```python
from build123d import *

# Parameters (mm, degrees)
CUT_EXTRUDE1_DEPTH       = 13.7
FILLET1_R                = 4
CIRPATTERN4_COUNT        = 6
FILLET1_OF_CIRPATTERN4_R = 4
CHAMFER1_SIZE            = 1
SKETCH9_R                = 83.55
SKETCH9_R_2              = 82.55
BOSS_EXTRUDE1_DEPTH      = 12.7


with BuildPart() as part:
    # Sketch2 → Revolve1 (revolve)
    with BuildSketch(Plane(origin=(0, 0, 0), x_dir=(0, 0, -1), z_dir=(1, 0, 0))):
        Polygon((-39.2125, 0), (-82.55, 0), (-82.55, 12.7), (-49.2125, 12.7), (-49.2125, 10), (-39.2125, 10), align=None)
    revolve(axis=Axis((0, -0.9525, 0), (0, 1, 0)))

    # Sketch8 → Cut-Extrude1 (cut, through all)
    with BuildSketch(Plane(origin=(0, 12.7, 0), x_dir=(1, 0, 0), z_dir=(0, 1, 0))):
        with BuildLine():
            Line((-34.364196, 69.520533), (-22.66059, 49.249293))
            ThreePointArc((-22.66059, 49.249293), (0, 54.2125), (22.66059, 49.249293))
            Line((22.66059, 49.249293), (34.364196, 69.520533))
            ThreePointArc((34.364196, 69.520533), (0, 77.55), (-34.364196, 69.520533))
        make_face()
    cut_extrude1 = extrude(amount=-CUT_EXTRUDE1_DEPTH, mode=Mode.SUBTRACT)

    # Fillet1
    fillet1_edges = [part.edges().sort_by_distance(p)[0] for p in [
        (22.66059, 6.35, -49.249293),
        (-22.66059, 6.35, -49.249293),
        (-34.364196, 6.35, -69.520533),
        (34.364196, 6.35, -69.520533),
    ]]
    fillet(fillet1_edges, radius=FILLET1_R)

    # CirPattern4: Cut-Extrude1 ×6 about axis
    cirpattern4_axis = Axis((0, 0, 0), (0, 1, 0))
    for i in range(1, CIRPATTERN4_COUNT):
        add(cut_extrude1.rotate(cirpattern4_axis, i * 360 / CIRPATTERN4_COUNT), mode=Mode.SUBTRACT)

    # Fillet1 of CirPattern4
    fillet1_of_cirpattern4_edges = [part.edges().sort_by_distance(p)[0] for p in [
        (-31.320844, 6.35, -44.249293),
        (-53.981433, 6.35, -5),
        (-77.388646, 6.35, -5),
        (-43.02445, 6.35, -64.520533),
        (-53.981433, 6.35, 5),
        (-31.320844, 6.35, 44.249293),
        (-43.02445, 6.35, 64.520533),
        (-77.388646, 6.35, 5),
        (-22.66059, 6.35, 49.249293),
        (22.66059, 6.35, 49.249293),
        (34.364196, 6.35, 69.520533),
        (-34.364196, 6.35, 69.520533),
        (31.320844, 6.35, 44.249293),
        (53.981433, 6.35, 5),
        (77.388646, 6.35, 5),
        (43.02445, 6.35, 64.520533),
        (53.981433, 6.35, -5),
        (31.320844, 6.35, -44.249293),
        (43.02445, 6.35, -64.520533),
        (77.388646, 6.35, -5),
    ]]
    fillet(fillet1_of_cirpattern4_edges, radius=FILLET1_OF_CIRPATTERN4_R)

    # Chamfer1
    chamfer1_edges = [part.edges().sort_by_distance(p)[0] for p in [
        (0, 12.7, -49.2125),
    ]]
    chamfer(chamfer1_edges, length=CHAMFER1_SIZE)

    # Sketch9 → Boss-Extrude1 (add)
    with BuildSketch(Plane.XZ):
        Circle(SKETCH9_R)
        Circle(SKETCH9_R_2, mode=Mode.SUBTRACT)
    extrude(amount=-BOSS_EXTRUDE1_DEPTH)


solid = part.part
```
Part model, mm, in its own coordinate system. A direction names the side the tool comes from. Round coordinates to 2 decimals unless told otherwise and drop trailing zeros. Loops run counter-clockwise (first coordinate to the right, second up) from the corner with the lowest first, then second, coordinate; pieces in that order, holes last. Notation, with made-up numbers: (80, -5.75) -> (112, -5.75) arc R20 ccw to (112, 25.25) -> close; hole circle Ø10 at (35.25, -28). An arc over 180 degrees is marked (long way). Use one line per item in the form item = value. Start each with the question number.
Item 1: Band-saw the part on B-B (z = 0). List the corners of the cut face in (x, y), plus the area to 3 significant figures.
Item 2: Two-plate mould, pull along X, no slides. Class faces 1 (the cylindrical face through (-22.256, 6.261, 50.523)), 2 (the flat face through (-38, 0, -12)): released by +X, released by -X, zero draft, split by the parting line, or undercut.
Item 3: Drop flat-ended pins along their axis: pin 1 Ø3 at (x, z) = (-9.5, -36) entering from -Y; pin 2 Ø1 at (x, y) = (3, 8.5) entering from +Z; pin 3 Ø4 at (x, y) = (-65, 7) entering from -Z; pin 4 Ø5 at (y, z) = (8, -43) entering from -X. Give the stop position or say it passes through.
Item 4: Band-saw the part on C-C (y = 5.5). Give the number of separate pieces and of enclosed holes in the cut face, plus the area to 3 significant figures.
Item 5: Band-saw the part on A-A (x = 0). List the corners of the cut face in (y, z).
Item 6: Tool access for faces 3 (the flat face through (-22, 10, -33)), 4 (the flat face through (-36.903, 6.439, -53.919)): list every direction of +Z, -Z, +X, -X, +Y, -Y with a clear straight run to the whole face (end or side of a thin tool).
Item 7: Drill centre lines: line 1 along X through (y, z) = (1.5, 35.5); line 2 along Z through (x, y) = (-13, 5); line 3 along X through (y, z) = (2.75, 56.5). Where is each one in solid material? Low to high.
Data:
q1.outline = (-83.55, 0) -> (-39.21, 0) -> (-39.21, 10) -> (-49.21, 10) -> (-49.21, 11.7) -> (-50.21, 12.7) -> (-83.55, 12.7) -> close; (39.21, 0) -> (83.55, 0) -> (83.55, 12.7) -> (50.21, 12.7) -> (49.21, 11.7) -> (49.21, 10) -> (39.21, 10) -> close
q1.area = 1,070 mm^2
q2.face_1 = undercut
q2.face_2 = zero draft
q3.pin_1 = through
q3.pin_2 = 83.51
q3.pin_3 = -54.88
q3.pin_4 = -73.08
q4.separate_pieces = 1
q4.enclosed_holes = 7
q4.area = 8,920 mm^2
q5.outline = (0, -83.55) -> (12.7, -83.55) -> (12.7, -77.55) -> (0, -77.55) -> close; (0, -54.21) -> (12.7, -54.21) -> (12.7, -50.21) -> (11.7, -49.21) -> (10, -49.21) -> (10, -39.21) -> (0, -39.21) -> close; (0, 39.21) -> (10, 39.21) -> (10, 49.21) -> (11.7, 49.21) -> (12.7, 50.21) -> (12.7, 54.21) -> (0, 54.21) -> close; (0, 77.55) -> (12.7, 77.55) -> (12.7, 83.55) -> (0, 83.55) -> close
q6.face_3 = +Y
q6.face_4 = +Y, -Y
q7.line_1 = -75.63 to -68.95, -40.97 to -16.65, 16.65 to 40.97, 68.95 to 75.63
q7.line_2 = -82.53 to -76.45, -52.63 to -36.99, 36.99 to 52.63, 76.45 to 82.53
q7.line_3 = -61.55 to -53.12, -38.39 to -26.85, 26.85 to 38.39, 53.12 to 61.55
